Part model, mm, in its own coordinate system. Give positions to 0.01 mm unless a question says otherwise; leave off trailing zeros. Write each loop counter-clockwise with the first axis right and the second up, starting at its lowest first coordinate (ties: lowest second). Pieces come first, ordered by that corner, then holes. Notation, with made-up numbers: (61, 71) - (83, 71) arc R25 cw to (83, 109) - close; hole circle Ø11 at (80, 26). An arc over 180 degrees is marked (long way). Answer in a Markdown table with one row per item. Add a question column.
1. Band-saw the part on C-C on y = 8. Write the cut outline in (x, z), plus the area to 3 significant figures.
2. Drop flat-ended pins along their axis: pin 1 Ø0.5 at (y, z) = (-8.5, 0.5) entering from +X; pin 2 Ø0.6 at (x, z) = (-8.5, 1.5) entering from -Y; pin 3 Ø4 at (x, y) = (10.5, -5.5) entering from -Z; pin 4 Ø3.5 at (x, y) = (-8, 0) entering from +Z. Give the stop position or say it passes through.
3. Band-saw the part on D-D on x = 0. Write the cut outline in (y, z) (3 decimals), plus the area to 3 significant figures.
4. Band-saw the part on A-A on y = 0. Write the cut outline in (x, z) (3 decimals), plus the area to 3 significant figures.
5. Probe line 1 along X through (y, z) = (-1, 0.95); line 2 along Y through (x, z) = (-8, 1.5) (3 decimals); line 3 along X through (y, z) = (-6, 0.95). List the from-to ranges inside material, lowest first.
6. Band-saw the part on B-B on x = 9.5. Write the cut outline in (y, z) (3 decimals), plus the area to 3 significant figures.
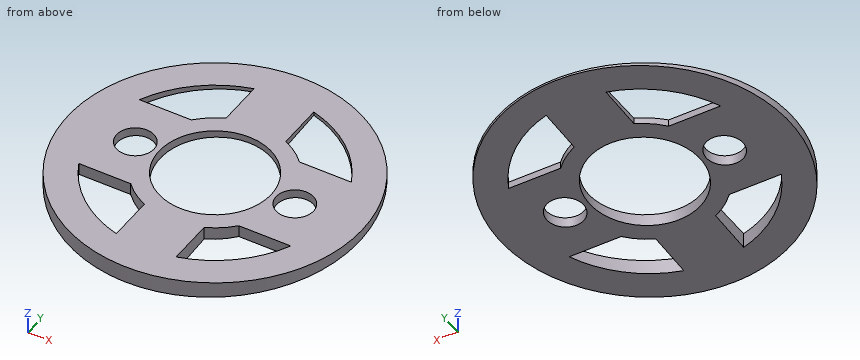
```python
from build123d import *

# Parameters (mm, degrees)
F0_R     = 14.75
F0_R_2   = 5.625
F1_DEPTH = 1.7
F2_D     = 3.75
F4_DEPTH = 15


with BuildPart() as f1:
    # F0 (on Top) → F1 (new body)
    with BuildSketch(Plane.XY):
        Circle(F0_R)
        with BuildLine():
            ThreePointArc((10.633085, 5), (11.467372, 2.561616), (11.75, 0))
            ThreePointArc((11.75, 0), (11.467372, -2.561616), (10.633085, -5))
            ThreePointArc((10.633085, -5), (7.521932, -9.026796), (3, -11.360568))
            ThreePointArc((3, -11.360568), (0, -11.75), (-3, -11.360568))
            ThreePointArc((-3, -11.360568), (-7.521932, -9.026796), (-10.633085, -5))
            ThreePointArc((-10.633085, -5), (-11.75, 0), (-10.633085, 5))
            ThreePointArc((-10.633085, 5), (-7.521932, 9.026796), (-3, 11.360568))
            ThreePointArc((-3, 11.360568), (0, 11.75), (3, 11.360568))
            ThreePointArc((3, 11.360568), (7.521932, 9.026796), (10.633085, 5))
        make_face(mode=Mode.SUBTRACT)
        with BuildLine():
            ThreePointArc((7.375, 0), (6.869236, 2.684069), (5.421312, 5))
            ThreePointArc((5.421312, 5), (4.299318, 5.992202), (3, 6.737256))
            ThreePointArc((3, 6.737256), (0, 7.375), (-3, 6.737256))
            ThreePointArc((-3, 6.737256), (-4.299318, 5.992202), (-5.421312, 5))
            ThreePointArc((-5.421312, 5), (-7.375, 0), (-5.421312, -5))
            ThreePointArc((-5.421312, -5), (-4.299318, -5.992202), (-3, -6.737256))
            ThreePointArc((-3, -6.737256), (0, -7.375), (3, -6.737256))
            ThreePointArc((3, -6.737256), (4.299318, -5.992202), (5.421312, -5))
            ThreePointArc((5.421312, -5), (6.869236, -2.684069), (7.375, 0))
        make_face()
        Circle(F0_R_2, mode=Mode.SUBTRACT)
        with BuildLine():
            Line((3, 6.737256), (3, 11.360568))
            ThreePointArc((3, 11.360568), (0, 11.75), (-3, 11.360568))
            Line((-3, 11.360568), (-3, 6.737256))
            ThreePointArc((-3, 6.737256), (0, 7.375), (3, 6.737256))
        make_face()
        with BuildLine():
            ThreePointArc((-3, -11.360568), (0, -11.75), (3, -11.360568))
            Line((3, -11.360568), (3, -6.737256))
            ThreePointArc((3, -6.737256), (0, -7.375), (-3, -6.737256))
            Line((-3, -6.737256), (-3, -11.360568))
        make_face()
        with BuildLine():
            ThreePointArc((10.633085, -5), (11.467372, -2.561616), (11.75, 0))
            ThreePointArc((11.75, 0), (11.467372, 2.561616), (10.633085, 5))
            Line((10.633085, 5), (5.421312, 5))
            ThreePointArc((5.421312, 5), (6.869236, 2.684069), (7.375, 0))
            ThreePointArc((7.375, 0), (6.869236, -2.684069), (5.421312, -5))
            Line((5.421312, -5), (10.633085, -5))
        make_face()
        with BuildLine():
            Line((-5.421312, 5), (-10.633085, 5))
            ThreePointArc((-10.633085, 5), (-11.75, 0), (-10.633085, -5))
            Line((-10.633085, -5), (-5.421312, -5))
            ThreePointArc((-5.421312, -5), (-7.375, 0), (-5.421312, 5))
        make_face()
    extrude(amount=F1_DEPTH)

    # F2 (through all)
    with Locations(Plane(origin=(0, 0, 0), x_dir=(1, 0, 0), z_dir=(0, 0, -1))):
        with Locations((-8, 0), (8, 0)):
            Hole(F2_D / 2)

    # F3 (on Right) → F4 (cut, symmetric)
    with BuildSketch(Plane.YZ):
        Polygon((14.75, 1.5), (-14.75, 0), (14.75, 0), align=None)
    extrude(amount=F4_DEPTH, both=True, mode=Mode.SUBTRACT)


solid = f1.part
```
Values:
| question | item | result |
|---|---|---|
| 1 | outline | (-12.39, 1.16) - (-8.61, 1.16) - (-8.61, 1.7) - (-12.39, 1.7) - close; (-3, 1.16) - (3, 1.16) - (3, 1.7) - (-3, 1.7) - close; (8.61, 1.16) - (12.39, 1.16) - (12.39, 1.7) - (8.61, 1.7) - close |
| 1 | area | 7.37 mm² |
| 2 | pin 1 | stops at x = 12.23 |
| 2 | pin 2 | stops at y = -12.26 |
| 2 | pin 3 | stops at z = 0.37 |
| 2 | pin 4 | passes through |
| 3 | outline | (-14.75, 0) - (-5.625, 0.464) - (-5.625, 1.7) - (-14.75, 1.7) - close; (5.625, 1.036) - (14.75, 1.5) - (14.75, 1.7) - (5.625, 1.7) - close |
| 3 | area | 17.3 mm² |
| 4 | outline | (-14.75, 0.75) - (-9.875, 0.75) - (-9.875, 1.7) - (-14.75, 1.7) - close; (-6.125, 0.75) - (-5.625, 0.75) - (-5.625, 1.7) - (-6.125, 1.7) - close; (5.625, 0.75) - (6.125, 0.75) - (6.125, 1.7) - (5.625, 1.7) - close; (9.875, 0.75) - (14.75, 0.75) - (14.75, 1.7) - (9.875, 1.7) - close |
| 4 | area | 10.2 mm² |
| 5 | line 1 | x = -14.72 to -9.59, -6.41 to -5.54, 5.54 to 6.41, 9.59 to 14.72 |
| 5 | line 2 | y = -12.392 to -8.606, -5 to -1.875, 1.875 to 5, 8.606 to 12.392 |
| 5 | line 3 | x = -13.47 to -10.1, -4.29 to 4.29, 10.1 to 13.47 |
| 6 | outline | (-11.283, 0.176) - (-6.915, 0.398) - (-6.915, 1.7) - (-11.283, 1.7) - close; (-5, 0.496) - (-1.125, 0.693) - (-1.125, 1.7) - (-5, 1.7) - close; (1.125, 0.807) - (5, 1.004) - (5, 1.7) - (1.125, 1.7) - close; (6.915, 1.102) - (11.283, 1.324) - (11.283, 1.7) - (6.915, 1.7) - close |
| 6 | area | 15.7 mm² |
